Verification items for the finished model (mm, model axes). A direction names the side the tool comes from. Round coordinates to 2 decimals unless told otherwise and drop trailing zeros. Order: outer loops, then holes, each group sorted by start corner. A loop starts at its lowest first (then second) coordinate and runs counter-clockwise, first axis right, second up. Notation, with made-up numbers: M -15,4.5 L 14,4.5 A12 ccw 14,23.5 Z; hole C -29.5,14.5 d1. An arc over 180 degrees is marked long. Return JSON: item names as keys, results as strings. Group by question number.
Autodesk Inventor part; units mm, degrees
ref_plane "YZ Plane" through (0, 0, 0) normal (1, 0, 0) x (0, 1, 0)
ref_plane "XZ Plane" through (0, 0, 0) normal (0, 1, 0) x (-1, 0, 0)
ref_plane "XY Plane" through (0, 0, 0) normal (0, 0, 1) x (1, 0, 0)
sketch "Эскиз1" plane through (0, 0, 0) normal (0, 0, 1) x (1, 0, 0)
  line L0 (0, 0) -> (0, 9.9999)
  line L1 (0, 9.9999) -> (27.2501, 9.9999)
  line L2 (27.2501, 9.9999) -> (29, 8.25)
  line L3 (29, 8.25) -> (35, 8.25)
  line L4 (35, 8.25) -> (35, 12.5)
  line L5 (35, 12.5) -> (39.3301, 20)
  line L6 (39.3301, 20) -> (60, 20)
  line L7 (60, 20) -> (60, 12)
  line L8 (60, 12) -> (99, 12)
  line L9 (99, 12) -> (99, 0)
  line L10 (99, 0) -> (0, 0)
  dimension "d1" = 45
  dimension "d2" = 30
  dimension "d3" = 6
  dimension "d4" = 35
  dimension "d7" = 24
  dimension "d8" = 19.9998
  dimension "d9" = 16.5
  dimension "d10" = 25
  dimension "d11" = 39
  dimension "d12" = 99
  dimension "d14" = 40
revolve "Вращение1" add sketch "Эскиз1" angle 360 about axis through (99, 0, 0) along (-1, 0, 0)
sketch "Эскиз2" plane through (99, 0, 0) normal (1, 0, 0) x (0, 0, -1)
  circle A0 centre (0, 0) radius 12
  line L0 (12, 0) -> (0, 12)
  line L1 (0, 12) -> (-12.0353, -0.0353)
  line L2 (-12.0353, -0.0353) -> (-0.0353, -12.0353)
  line L3 (-0.0353, -12.0353) -> (12, 0)
extrude "Выдавливание1" [suppressed]
sketch "Эскиз3" plane through (0, 0, 0) normal (0, 1, 0) x (-1, 0, 0)
  point P0 (0, 0)
sketch "Эскиз4" plane through (0, 0, 0) normal (0, 1, 0) x (-1, 0, 0)
  line L0 (-60, -12) -> (-99, -12)
  line L1 (-66, -12) -> (-86, -12)
  line L2 (-86, -12) -> (-86, -6.1869)
  line L3 (-86, -6.1869) -> (-66, -6.1869)
  line L4 (-66, -6.1869) -> (-66, -12)
  line L5 (-60, 12) -> (-99, 12)
  line L6 (-66, 12) -> (-86, 12)
  line L7 (-86, 12) -> (-86, 5.8131)
  line L8 (-86, 5.8131) -> (-66, 5.8131)
  line L9 (-66, 5.8131) -> (-66, 12)
  line L10 (-60, 20) -> (-60, -20)
  point P0 (0, 0)
  dimension "d18" = 6
  dimension "d19" = 6
  dimension "d20" = 20
  dimension "d21" = 12
extrude "Выдавливание2" cut sketch "Эскиз4" along normal through all both and the other way through all
sketch "Эскиз5" plane through (0, 0, 0) normal (0, 0, 1) x (1, 0, 0)
  line L0 (60, -12) -> (60, 12)
  line L1 (60, -20) -> (60, 20)
  line L2 (-21.8, 0) -> (130.8, 0)
  circle A0 centre (72, 0) radius 3
  point P0 (0, 0)
  dimension "d24" = 6
  dimension "d25" = 12
extrude "Выдавливание3" cut sketch "Эскиз5" along normal through all both and the other way through all
thread "Резьба1"
chamfer "Фаска1" distance 2.5 angle 45 1 edges at (0, -9.9999, 0)
fillet "Сопряжение1" radius 1 1 edges at (29, -8.25, 0)
fillet "Сопряжение2" radius 1.6 1 edges at (35, -8.25, 0)
sketch "Эскиз6" plane through (72, 0, 0) normal (0, 0, 1) x (1, 0, 0)
  point P0 (-72, 0)
sketch "Эскиз7" plane through (99, -8.4853, 8.4853) normal (0, 0, 1) x (1, 0, 0)
  point P0 (-99, 8.4853)
sketch "Эскиз8" plane through (99, 0, 0) normal (1, 0, 0) x (0, 0, -1)
  circle A0 centre (0, 0) radius 12
  circle A1 centre (0, 0) radius 12
  line L0 (12, -0.0264) -> (0, 12)
  line L1 (0, 12) -> (-12, 0.0264)
  line L2 (-12, 0.0264) -> (0, -12)
  line L3 (0, -12) -> (12, -0.0264)
extrude "Выдавливание4" add sketch "Эскиз8" along normal blind 16 contours L0 L3 L2 L1
properties part number "Семинр Курганова вал"
1. Go/stop test with flat-tipped pins: pin 1 (6 mm diameter, centred on x = 34.5, z = 11.5, fed in from +Y); pin 2 (10 mm diameter, centred on y = -16, z = 15.5, fed in from +X); pin 3 (5 mm diameter, centred on x = 64, y = -5, fed in from +Z); pin 4 (4 mm diameter, centred on x = 29, y = 12, fed in from -Z). Record where each tip stops, or that it passes through.
2. Access from +Z, -Z, +X, -X, +Y, -Y to the whole of each face (thin tool, end or side, straight path). Record for faces 1 (the face through (106.888, 5.903, -6.084)), 2 (the face through (86, 0, -8)), 3 (the face through (66, 0, 8)).
3. Cross-section at C-C (x = 93). Enter the section's corners in (y, z).
4. Cross-section at A-A (x = 72). Enter the section's corners in (y, z), plus the area to 3 significant figures.
5. Draft check along X on faces 4 (the face through (99, 7, -7)), 5 (the face through (15.05, 9.54, 3)), 6 (the face through (69.6, -1.8, -0.1)). Enter one of: +X half, -X half, draft (parallel to the pull), parting line (faces both ways), or undercut.
6. Thickness scan on line 1 along X through (y, z) = (0, -3.25); line 2 along X through (y, z) = (-7, 7); line 3 along Z through (x, y) = (85, 1.5). Record the ranges inside material, lowest first. Write a range as from..to.
7. Cross-section at B-B (x = 20.5). Enter the section's corners in (y, z), plus the area to 3 significant figures.
Computed:
{
 "1": {"pin 1": "stops at y = 12.77", "pin 2": "stops at x = 60", "pin 3": "stops at z = 11.74", "pin 4": "passes through"},
 "2": {"face 1": "-Z, +X, +Y", "face 2": "-Z, +Y, -Y", "face 3": "+Z, +Y, -Y"},
 "3": {"outline": "C 0,0 d24"},
 "4": {"outline": "M -10.5,5.81 A12 ccw -10.28,-6.19 L -3,-6.19 L -3,5.81 Z; M 3,-6.19 L 10.28,-6.19 A12 ccw 10.5,5.81 L 3,5.81 Z", "area": "203 mm²"},
 "5": {"face 4": "+X half", "face 5": "draft", "face 6": "undercut"},
 "6": {"line 1": "x = 0..69, 75..115", "line 2": "x = 2.4..27.35, 35..66, 86..99", "line 3": "z = -6.19..5.81"},
 "7": {"outline": "C 0,0 d20", "area": "314 mm²"}
}
